Geometry check sheet. Reference: the model listing, model coordinates, mm. Round coordinates to 2 decimals unless told otherwise and drop trailing zeros. Loops run counter-clockwise (first coordinate to the right, second up) from the corner with the lowest first, then second, coordinate; pieces in that order, holes last. Notation, with made-up numbers: (31, 36) - (72, 36) arc R36 ccw to (72, 72) - close; hole circle Ø4 at (63, 2.5). An arc over 180 degrees is marked (long way). Answer in a Markdown table with one row per item. Add a question column.
```python
from build123d import *

# Parameters (mm, degrees)
SKETCH1_W           = 180
SKETCH1_H           = 70
SKETCH1_R           = 9
BOSS_EXTRUDE1_DEPTH = 5


with BuildPart() as part:
    # Sketch1 → Boss-Extrude1 (new, symmetric)
    with BuildSketch(Plane.XY):
        Rectangle(SKETCH1_W, SKETCH1_H)
        with Locations((60, 0)):
            Circle(SKETCH1_R, mode=Mode.SUBTRACT)
        with Locations((-40, 0)):
            Circle(SKETCH1_R, mode=Mode.SUBTRACT)
    extrude(amount=BOSS_EXTRUDE1_DEPTH, both=True)


solid = part.part
```
Q1. Cross-section at C-C, the plane z = 3. Enter the section's corners in (x, y), plus the area to 3 significant figures.
Q2. Cross-section at B-B, the plane y = 0. Enter the section's corners in (x, z).
Q3. Scan lines: line 1 (Y direction, x = -40, z = -2.25); line 2 (X direction, y = 2, z = 0); line 3 (Y direction, x = 57, z = 3.75). Record each from-to range of solid material in increasing order. Write a range as from..to.
Q4. Cross-section at A-A, the plane x = -40. Enter the section's corners in (y, z).
Q5. Release check for a two-part mould opening along X. For faces 1 (the flat face through (90, 0, 0)), 2 (the cylindrical face through (68.584, 2.703, -0.07)), 3 (the flat face through (-1, -35, 0)) record: +X half, -X half, draft (parallel to the pull), parting line (faces both ways), or undercut.
Check sheet entries:
| question | item | result |
|---|---|---|
| 1 | outline | (-90, -35) - (90, -35) - (90, 35) - (-90, 35) - close; hole circle Ø18 at (-40, 0); hole circle Ø18 at (60, 0) |
| 1 | area | 12,100 mm² |
| 2 | outline | (-90, -5) - (-49, -5) - (-49, 5) - (-90, 5) - close; (-31, -5) - (51, -5) - (51, 5) - (-31, 5) - close; (69, -5) - (90, -5) - (90, 5) - (69, 5) - close |
| 3 | line 1 | -35..-9, 9..35 |
| 3 | line 2 | -90..-48.77, -31.23..51.23, 68.77..90 |
| 3 | line 3 | -35..-8.49, 8.49..35 |
| 4 | outline | (-35, -5) - (-9, -5) - (-9, 5) - (-35, 5) - close; (9, -5) - (35, -5) - (35, 5) - (9, 5) - close |
| 5 | face 1 | +X half |
| 5 | face 2 | undercut |
| 5 | face 3 | draft |
